Solid Edge part; units mm, degrees
sketch "Sketch1" plane through (0, 0, 0) normal (0, -1, 0) x (1, 0, 0)
  line L0 (-20, -20) -> (20, -20)
  line L1 (20, -20) -> (20, 20)
  line L2 (20, 20) -> (-20, 20)
  line L3 (-20, 20) -> (-20, -20)
  line L4 (-25, -25) -> (25, -25)
  line L5 (25, -25) -> (25, 25)
  line L6 (25, 25) -> (-25, 25)
  line L7 (-25, 25) -> (-25, -25)
  dimension "D1" = 20
extrude "Protrusion1" add sketch "Sketch1" along normal blind 5
sketch "Sketch2" plane through (0, 0, 0) normal (0, 1, 0) x (-1, 0, 0)
  line L0 (-25, -25) -> (25, -25)
  line L1 (25, -25) -> (25, 25)
  line L2 (25, 25) -> (-25, 25)
  line L3 (-25, 25) -> (-25, -25)
  circle A0 centre (17, 17) radius 0.9
  circle A1 centre (-17, 17) radius 0.9
  circle A2 centre (-17, -17) radius 0.9
  circle A3 centre (17, -17) radius 0.9
extrude "Extrusionsausprägung_2" add sketch "Sketch2" along normal blind 8
sketch "Sketch3" plane through (-25, 1.5, 0) normal (-1, 0, 0) x (0, -1, 0)
  line L0 (6.5, 25) -> (-6.5, 25)
  arc A0 (20.0295, 49.1481) -> (-6.5, 25) centre (30.1482, 11.3846) ccw
  line L1 (20.0295, 49.1481) -> (21.3236, 44.3185)
  arc A1 (21.3236, 44.3185) -> (6.5, 25) centre (26.5, 25) ccw
  line L2 (6.5, -25) -> (-6.5, -25)
  arc A2 (-6.5, -25) -> (20.0295, -49.1481) centre (30.1482, -11.3846) ccw
  line L3 (21.3236, -44.3185) -> (20.0295, -49.1481)
  arc A3 (6.5, -25) -> (21.3236, -44.3185) centre (26.5, -25) ccw
  dimension "D1" = 20.0295
  dimension "D2" = 21.3236
extrude "Protrusion2" add sketch "Sketch3" against normal up to vertex (50 mm away)
sketch "Sketch4" plane through (0, -5, 0) normal (0, -1, 0) x (1, 0, 0)
  line L0 (-25, 14) -> (-25, -14)
  line L1 (-25, -14) -> (-14, -14)
  line L2 (-14, -14) -> (-14, -20)
  line L3 (-14, -20) -> (14, -20)
  line L4 (14, -20) -> (14, -14)
  line L5 (14, -14) -> (20, -14)
  line L6 (20, -14) -> (20, 14)
  line L7 (20, 14) -> (14, 14)
  line L8 (14, 14) -> (14, 20)
  line L9 (14, 20) -> (-14, 20)
  line L10 (-14, 20) -> (-14, 14)
  line L11 (-14, 14) -> (-25, 14)
  dimension "D1" = 14
extrude "Extrusionsausschnitt_1" cut sketch "Sketch4" against normal blind 10
sketch "Sketch5" plane through (0, 8, 0) normal (0, 1, 0) x (-1, 0, 0)
  line L0 (-7.5, -25) -> (7.5, -25)
  line L1 (7.5, -25) -> (7.5, 25)
  line L2 (7.5, 25) -> (-7.5, 25)
  line L3 (-7.5, 25) -> (-7.5, -25)
  dimension "D1" = 7.5
extrude "Extrusionsausprägung_6" add sketch "Sketch5" along normal blind 40
sketch "Sketch6" plane through (-7.5, 28, 0) normal (-1, 0, 0) x (0, -1, 0)
  line L0 (20, -6.3116) -> (20, -25)
  line L1 (-8.5148, -26.2779) -> (20, -6.3116)
  line L2 (-17.1184, -13.9906) -> (-8.5148, -26.2779)
  line L3 (20, 12) -> (-17.1184, -13.9906)
  line L4 (20, 25) -> (20, 12)
  line L5 (-20, 25) -> (20, 25)
  line L6 (-20, 25) -> (-40.7628, -3.883)
  line L7 (-40.7628, -3.883) -> (-20, -25)
  line L8 (-20, -25) -> (-14.3498, -34.4374)
  line L9 (-14.3498, -34.4374) -> (20, -25)
  dimension "D1" = 17.1184
  dimension "D2" = 20
extrude "Cutout1" cut sketch "Sketch6" against normal through all
properties material "Nylon, allgemein"
Design review of the part built by this model. Coordinates are the model's own, in mm. A direction names the side the tool comes from. Round coordinates to 2 decimals unless told otherwise and drop trailing zeros. Order: outer loops, then holes, each group sorted by start corner. A loop starts at its lowest first (then second) coordinate and runs counter-clockwise, first axis right, second up. Notation, with made-up numbers: M 37,-14 L 53,-14 A27 cw 53,21 Z; hole C 0.25,36.25 d10. An arc over 180 degrees is marked long. Answer as CSV lines item,"result". Start each with the question number.
1) Add section C-C (y = -12.5). Give the boundary of the cut face in (x, z), then the cut area to 3 significant figures.
2) Tool access review of faces 1 (the face through (20.5, -5, 3.8)), 2 (the face through (-0.35, -2.525, 40.472)), 3 (the face through (0, 0, -20)), 4 (the face through (17, 2, 14)), 5 (the face through (-0.35, -2.14, -40.12)): name each direction out of +Z, -Z, +X, -X, +Y, -Y from which nothing blocks a thin tool from reaching the whole face with its end or side.
3) Add section A-A (z = -22). Give the boundary of the cut face in (x, y), then the cut area to 3 significant figures.
4) For pin 1 Ø1.8 at (x, z) = (17.5, 16.5) entering from -Y; pin 2 Ø2 at (x, z) = (17, 17) entering from +Y; pin 3 Ø1 at (x, z) = (9, 24.5) entering from -Y, all flat-tipped, find the tip position at first contact; note any pin that passes through.
5) Wall thickness on line 1 along Z through (x, y) = (-17, 3); line 2 along Z through (x, y) = (17, 4); line 3 along Z through (x, y) = (17, 5.5): over which ranges is each line inside the solid? List them lowest first. Write a range as [from, to].
6) Add section D-D (z = 5). Give the boundary of the cut face in (x, y).
7) The part is to be moulded in two halves that separate along X. For faces 6 (the face through (-21, 1, 14)), 7 (the face through (25, -3, -1)), 8 (the face through (-14, 2, -17)), say which applies: +X half, -X half, draft (parallel to the pull), parting line (faces both ways), or undercut.
8) Add section B-B (x = -10.5). Give the boundary of the cut face in (y, z).
Resolved:
1,outline,"M -25,-46.99 L 25,-46.99 L 25,-40.61 L -25,-40.61 Z; M -25,40.61 L 25,40.61 L 25,46.99 L -25,46.99 Z"
1,area,"638 mm^2"
2,face 1,"+X, -X, -Y"
2,face 2,"+Z, +X, -X, +Y"
2,face 3,"-Y"
2,face 4,"-X, -Y"
2,face 5,"-Z, +X, -X, +Y"
3,outline,"M -25,-5 L 25,-5 L 25,8 L -25,8 Z; M -7.5,30.41 L 7.5,30.41 L 7.5,39.51 L -7.5,39.51 Z"
3,area,"787 mm^2"
4,pin 1,"y = 0"
4,pin 2,"y = 8"
4,pin 3,"y = -5"
5,line 1,"[-34.34, -17.9], [-16.1, -14], [14, 16.1], [17.9, 34.34]"
5,line 2,"[-32.89, -17.9], [-16.1, -14], [14, 16.1], [17.9, 32.89]"
5,line 3,"[-30.42, -17.9], [-16.1, 16.1], [17.9, 30.42]"
6,outline,"M -25,5 L 20,5 L 20,-5 L 25,-5 L 25,8 L 7.5,8 L 7.5,18 L -7.5,18 L -7.5,8 L -25,8 Z"
7,face 6,"draft"
7,face 7,"+X half"
7,face 8,"undercut"
8,outline,"M -19.82,-44.32 L -18.53,-49.15 A39.1 ccw 8,-25 L 8,25 A39.1 ccw -18.53,49.15 L -19.82,44.32 A20 cw -5,25 L -5,20 L 5,20 L 5,-20 L -5,-20 L -5,-25 A20 cw Z"
